from build123d import *

# Parameters (mm, degrees)
DODANIE_WYCI_GNI_CIE1_DEPTH = 15
SKORUPA1_T                  = 3


with BuildPart() as part:
    # Szkic1 → Dodanie-wyciągnięcie1 (new body)
    with BuildSketch(Plane(origin=(0, 0, 0), x_dir=(1, 0, 0), z_dir=(0, 1, 0))):
        Polygon((0, 0), (454, 0), (454, 220), (484, 220), (484, 409), (0, 409), align=None)
    extrude(amount=-DODANIE_WYCI_GNI_CIE1_DEPTH)

    # Skorupa1
    skorupa1_openings = [part.faces().sort_by_distance(p)[0] for p in [
        (234.170613934, -15, -207.75936997),
    ]]
    offset(amount=SKORUPA1_T, openings=skorupa1_openings, kind=Kind.INTERSECTION)


solid = part.part
Work out the finished part from the listing and answer in its coordinate system (mm). A direction names the side the tool comes from. Give positions to 0.01 mm unless a question says otherwise; leave off trailing zeros. Order: outer loops, then holes, each group sorted by start corner. A loop starts at its lowest first (then second) coordinate and runs counter-clockwise, first axis right, second up. Notation, with made-up numbers: (-16, 2.25) -> (23, 2.25) arc R36 cw to (23, 36.25) -> close; hole circle Ø9 at (37.5, 77.5). An arc over 180 degrees is marked (long way). Answer as a JSON object with one key per item and string values. Group by question number.
1. Section B-B on z = -278.5 is taken. Determine the outline of the cut face in (x, y), plus the area to 3 significant figures.
2. The mould has two halves that part along X. Classify faces 1 (the flat face through (457, -6, -105)), 2 (the flat face through (-3, -6, -207)), 3 (the flat face through (245, -6, -412)), 4 (the flat face through (0, -7, -207)): released by +X, released by -X, zero draft, split by the parting line, or undercut.
3. Consider line 1 along X through (y, z) = (-4.5, -173.5); line 2 along Z through (x, y) = (200, -5.5); line 3 along X through (y, z) = (-4.25, -338.5). Determine where each line is inside the solid, lowest interval first. Write a range as [from, to].
4. Section C-C on x = 95.5 is taken. Determine the outline of the cut face in (y, z), plus the area to 4 significant figures.
5. A flat-ended cylindrical pin translates along its axis: pin 1 Ø4.5 at (y, z) = (-11, -104) entering from +X. Find the tip coordinate at first contact, or state that the pin passes through.
6. Section A-A on y = -6.25 is taken. Determine the outline of the cut face in (x, z).
7. A tool of negligible diameter and unlimited length cuts with its end or side. For faces 5 (the flat face through (245, -7, -409)), 6 (the flat face through (224, -6, 3)), 7 (the flat face through (472, -6, -217)), from which of +Z, -Z, +X, -X, +Y, -Y can it reach the whole face along a straight path? Write none if from no direction.
Result sheet:
{
 "1": {"outline": "(-3, -15) -> (0, -15) -> (0, 0) -> (484, 0) -> (484, -15) -> (487, -15) -> (487, 3) -> (-3, 3) -> close", "area": "1,560 mm^2"},
 "2": {"face 1": "released by +X", "face 2": "released by -X", "face 3": "zero draft", "face 4": "undercut"},
 "3": {"line 1": "x = [-3, 0], [454, 457]", "line 2": "z = [-412, -409], [0, 3]", "line 3": "x = [-3, 0], [484, 487]"},
 "4": {"outline": "(-15, -412) -> (3, -412) -> (3, 3) -> (-15, 3) -> (-15, 0) -> (0, 0) -> (0, -409) -> (-15, -409) -> close", "area": "1,335 mm^2"},
 "5": {"pin 1": "stops at x = 457"},
 "6": {"outline": "(-3, -412) -> (487, -412) -> (487, -217) -> (457, -217) -> (457, 3) -> (-3, 3) -> close; hole (0, -409) -> (484, -409) -> (484, -220) -> (454, -220) -> (454, 0) -> (0, 0) -> close"},
 "7": {"face 5": "-Y", "face 6": "+Z, +X, -X, +Y, -Y", "face 7": "+Z, +X, +Y, -Y"}
}
